Study the drawing (mm; zero at the part's minimum x, y, z) and answer. Coordinates: 2 decimals unless noted, no trailing zeros. Loops run counter-clockwise (first coordinate to the right, second up) from the corner with the lowest first, then second, coordinate; pieces in that order, holes last. Notation, with made-up numbers: (53.5, 44.25) - (85.5, 44.25) arc R11 ccw to (85.5, 53.25) - close; hole circle Ø5 at (12, 82.5). An arc over 180 degrees is marked (long way). One line per item, written item: value. Start each with the question number.
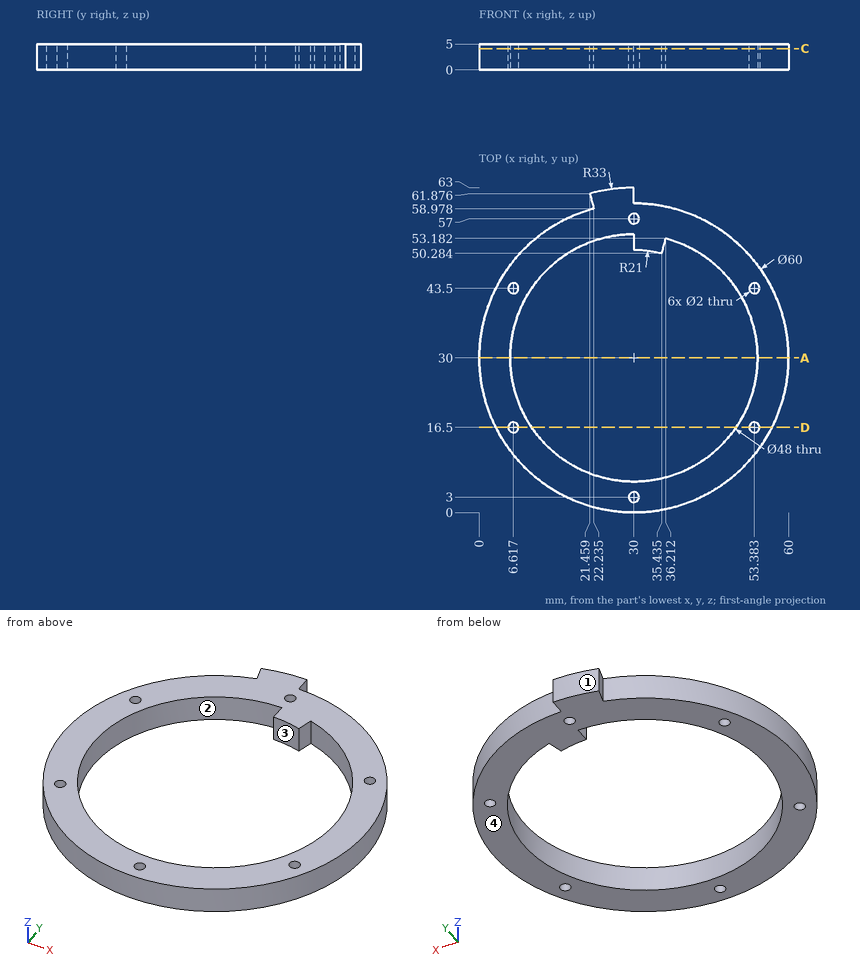
1) Straight lines are drawn through the part: L1, parallel to X at y = 43.5, z = 2.35 (1 decimal); L2, parallel to X at y = 30, z = 2.45; L3, parallel to Y at x = 14.5, z = 4.5 (1 decimal). For each, find the intervals that lie inside material, in ascending order.
2) Section D-D, the plane y = 16.5 is taken. Determine the outline of the cut face in (x, z).
3) Flat-ended cylindrical pins translate along their axes: P1, Ø2.5, axis at y = 52, z = 2, coming from the -X side (1 decimal); P2, Ø3, axis at x = 24, z = 1, coming from the +Y side; P3, Ø1.5, axis at x = 13, z = 1, coming from the +Y side. Find the tip coordinate at first contact, or state that the pin passes through.
4) Section A-A, the plane y = 30 is taken. Determine the outline of the cut face in (x, z).
5) Section C-C, the plane z = 4.1 is taken. Determine the outline of the cut face in (x, y) (1 decimal).
6) Determine the mould class of the marked faces 1, 2, 3 and 4 for opening direction Y: released by +Y, released by -Y, zero draft, split by the parting line, or undercut.
Answer below:
1. L1: 3.2 to 5.6, 7.6 to 10.2, 49.8 to 52.4, 54.4 to 56.8
1. L2: 0 to 6, 54 to 60
1. L3: 4.3 to 11.7, 48.3 to 55.7
2. outline: (3.21, 0) - (5.62, 0) - (5.62, 5) - (3.21, 5) - close; (7.62, 0) - (10.16, 0) - (10.16, 5) - (7.62, 5) - close; (49.84, 0) - (52.38, 0) - (52.38, 5) - (49.84, 5) - close; (54.38, 0) - (56.79, 0) - (56.79, 5) - (54.38, 5) - close
3. P1: x = 8.3
3. P2: y = 62.69
3. P3: y = 55.22
4. outline: (0, 0) - (6, 0) - (6, 5) - (0, 5) - close; (54, 0) - (60, 0) - (60, 5) - (54, 5) - close
5. outline: (21.5, 61.9) - (22.2, 59) arc R30 ccw (long way) to (30, 60) - (30, 63) arc R33 ccw to start; hole circle Ø2 at (6.6, 16.5); hole circle Ø2 at (6.6, 43.5); hole circle Ø2 at (30, 3); hole circle Ø2 at (30, 57); hole (30, 51) - (30, 54) arc R24 ccw (long way) to (36.2, 53.2) - (35.4, 50.3) arc R21 ccw to start; hole circle Ø2 at (53.4, 16.5); hole circle Ø2 at (53.4, 43.5)
6. face 1: released by +Y
6. face 2: undercut
6. face 3: undercut
6. face 4: zero draft
